```python
from build123d import *

# Parameters (mm, degrees)
SKETCH_W  = 50.7
SKETCH_H  = 31.3
PAD_DEPTH = 3.5
FILLET_R  = 2


with BuildPart() as part:
    # Sketch → Pad (new body)
    with BuildSketch(Plane.XY):
        Rectangle(SKETCH_W, SKETCH_H)
        with BuildLine():
            Line((-17.738958, 9), (17.738958, 9))
            ThreePointArc((18.7, 8.000759), (19.459707, 9.693196), (17.738958, 9))
            Line((18.7, 8.000759), (18.7, -8.000759))
            ThreePointArc((17.738958, -9), (19.459707, -9.693196), (18.7, -8.000759))
            Line((17.738958, -9), (-17.738958, -9))
            ThreePointArc((-18.7, -8.000759), (-19.459707, -9.693196), (-17.738958, -9))
            Line((-18.7, -8.000759), (-18.7, 7.61377))
            ThreePointArc((-17.738958, 9), (-19.482861, 9.182759), (-18.7, 7.61377))
        make_face(mode=Mode.SUBTRACT)
    extrude(amount=PAD_DEPTH)

    # Fillet
    fillet_edges = [part.edges().sort_by_distance(p)[0] for p in [
        (25.35, 15.65, 1.75),
        (25.35, -15.65, 1.75),
        (-25.35, -15.65, 1.75),
        (-25.35, 15.65, 1.75),
    ]]
    fillet(fillet_edges, radius=FILLET_R)


solid = part.part
```
Source: CAD feature listing. Evaluate the final solid. Frame: model axes, mm. A direction names the side the tool comes from. Give positions to 0.01 mm unless a question says otherwise; leave off trailing zeros. Order: outer loops, then holes, each group sorted by start corner. A loop starts at its lowest first (then second) coordinate and runs counter-clockwise, first axis right, second up.
(1) Contact query for a flat-ended pin moving along its axis: P1, Ø1.6, axis at x = 18.74, y = -9, coming from the +Z side. Output: stop coordinate, or through.
(2) Pull-direction query (X, two-part tool) for faces 3 (the face through (25.35, 0, 2)), 4 (the face through (-25.35, 0, 2)), 5 (the face through (0, -9, 2)); classes: +X half, -X half, draft (parallel to the pull), parting line (faces both ways), or undercut.
(3) Section query C-C (y = 3). Return the cut outline in (x, z).
(4) Access query for faces 1 (the face through (0, 9, 2)), 2 (the face through (0, 15.65, 2)). Directions: +Z, -Z, +X, -X, +Y, -Y. A direction counts if a zero-diameter tool reaches every point of the face in a straight line with its end or side. Return the directions, or none.
(5) Material intervals for line 1 along Y through (x, z) = (-11, 2.65); line 2 along X through (y, z) = (0, 1.6); line 3 along X through (y, z) = (-9.5, 1.5), sorted ascending.
(6) Section query A-A (z = 2.6). Return the cut outline in (x, y).
(7) Section query B-B (x = -1). Return the cut outline in (y, z), plus the area to 4 significant figures.
Outcome:
1. P1: passes through
2. face 3: +X half
2. face 4: -X half
2. face 5: undercut
3. outline: (-25.35, 0) - (-18.7, 0) - (-18.7, 3.5) - (-25.35, 3.5) - close; (18.7, 0) - (25.35, 0) - (25.35, 3.5) - (18.7, 3.5) - close
4. face 1: +Z, -Z
4. face 2: +Z, -Z, +X, -X, +Y
5. line 1: y = -15.65 to -9, 9 to 15.65
5. line 2: x = -25.35 to -18.7, 18.7 to 25.35
5. line 3: x = -25.35 to -19.6, -17.87 to 17.87, 19.6 to 25.35
6. outline: (-25.35, -13.65) arc R2 ccw to (-23.35, -15.65) - (23.35, -15.65) arc R2 ccw to (25.35, -13.65) - (25.35, 13.65) arc R2 ccw to (23.35, 15.65) - (-23.35, 15.65) arc R2 ccw to (-25.35, 13.65) - close; hole (-18.7, -8) arc R1 ccw (long way) to (-17.74, -9) - (17.74, -9) arc R1 ccw (long way) to (18.7, -8) - (18.7, 8) arc R1 ccw (long way) to (17.74, 9) - (-17.74, 9) arc R1 ccw (long way) to (-18.7, 7.61) - close
7. outline: (-15.65, 0) - (-9, 0) - (-9, 3.5) - (-15.65, 3.5) - close; (9, 0) - (15.65, 0) - (15.65, 3.5) - (9, 3.5) - close
7. area: 46.55 mm2
